Geometry: final body of the model. Coordinates: model frame, mm. Face numbers are marked on the shaded views. A direction names the side the tool comes from. Round coordinates to 2 decimals unless told otherwise and drop trailing zeros. Order: outer loops, then holes, each group sorted by start corner. A loop starts at its lowest first (then second) coordinate and runs counter-clockwise, first axis right, second up. Notation, with made-up numbers: M 63.5,50 L 100.5,50 A14 ccw 100.5,61 Z; hole C 22,-26.75 d10. An arc over 180 degrees is marked long. Return JSON: item names as keys, results as strings. Group by question number.
Q1. Mould query, pull axis X, two halves, no side actions, for the marked faces 6, 7, 8 and 9. Classes: released by +X, released by -X, zero draft, split by the parting line, or undercut.
Q2. Access query for the marked faces 1, 2, 3, 4 and 5. Directions: +Z, -Z, +X, -X, +Y, -Y. A direction counts if a zero-diameter tool reaches every point of the face in a straight line with its end or side. Return the directions, or none.
Q3. Contact query for flat-ended pins moving along their axis: pin 1 (4 mm diameter, centred on x = -90, z = -27, fed in from -Y); pin 2 (6 mm diameter, centred on x = -89.5, z = -37, fed in from +Y). Output: stop coordinate, or through.
Q4. Cut plane D-D on y = 25.5. Output: boundary loops of the cut face in (x, z).
Q5. Ray query, probe 1 along X at (y, z) = (-4, -21); probe 2 along Y at (x, z) = (-28, -14); probe 3 along Z at (x, y) = (-60, -7). Return the intervals inside material, ascending.
Q6. Cut plane C-C on x = -81.5. Output: boundary loops of the cut face in (y, z), and give its area (3 significant figures).
Q7. Cut plane B-B on y = 11. Output: boundary loops of the cut face in (x, z), and give its area (3 significant figures).
Q8. Cut plane A-A on z = -6. Output: boundary loops of the cut face in (x, y).
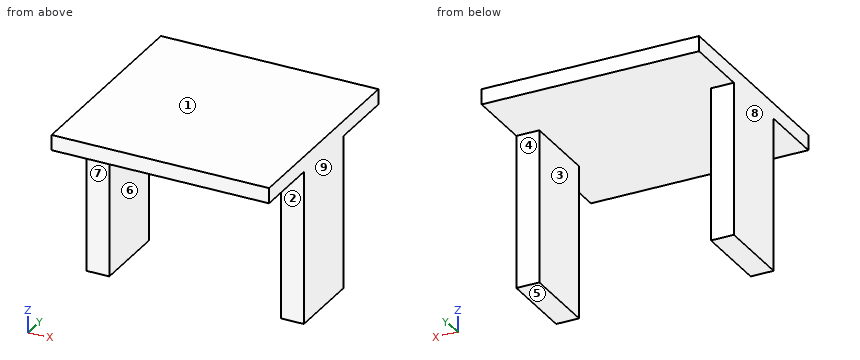
```python
from build123d import *

# Parameters (mm, degrees)
F0_W     = 72.225
F0_H     = 69.85
F1_DEPTH = 5.08
F3_DEPTH = 50.8


with BuildPart() as f1:
    # F0 (on Top) → F1 (new body)
    with BuildSketch(Plane.XY):
        with Locations((-58.976147, 0.364591)):
            Rectangle(F0_W, F0_H)
    extrude(amount=F1_DEPTH)

    # F2 (on face) → F3 (join)
    with BuildSketch(Plane(origin=(0, 0, 0), x_dir=(1, 0, 0), z_dir=(0, 0, -1))):
        Polygon((-95.088647, 12.335409), (-95.088647, -0.364591), (-95.088647, -13.064591), (-87.468647, -13.064591), (-87.468647, 12.335409), align=None)
        Polygon((-22.863647, -0.364591), (-22.863647, 12.335409), (-30.483647, 12.335409), (-30.483647, -13.064591), (-22.863647, -13.064591), align=None)
    extrude(amount=F3_DEPTH)


solid = f1.part
```
Result sheet:
{
 "1": {"face 6": "undercut", "face 7": "zero draft", "face 8": "released by -X", "face 9": "released by +X"},
 "2": {"face 1": "+Z, +X, -X, +Y, -Y", "face 2": "-Z, +X, -X, -Y", "face 3": "-Z, +Y, -Y", "face 4": "-Z, +X, -X, +Y", "face 5": "-Z, +X, -X, +Y, -Y"},
 "3": {"pin 1": "stops at y = -12.34", "pin 2": "stops at y = 13.06"},
 "4": {"outline": "M -95.09,0 L -22.86,0 L -22.86,5.08 L -95.09,5.08 Z"},
 "5": {"probe 1": "x = -95.09 to -87.47, -30.48 to -22.86", "probe 2": "y = -12.34 to 13.06", "probe 3": "z = 0 to 5.08"},
 "6": {"outline": "M -34.56,0 L 35.29,0 L 35.29,5.08 L -34.56,5.08 Z", "area": "355 mm²"},
 "7": {"outline": "M -95.09,-50.8 L -87.47,-50.8 L -87.47,0 L -30.48,0 L -30.48,-50.8 L -22.86,-50.8 L -22.86,5.08 L -95.09,5.08 Z", "area": "1,140 mm²"},
 "8": {"outline": "M -95.09,-12.34 L -87.47,-12.34 L -87.47,13.06 L -95.09,13.06 Z; M -30.48,-12.34 L -22.86,-12.34 L -22.86,13.06 L -30.48,13.06 Z"}
}
